from build123d import *

# Parameters (mm, degrees)
BOSS_EXTRUDE1_DEPTH = 4
BOSS_EXTRUDE2_DEPTH = 31
CHAMFER2_SIZE       = 31
CUT_EXTRUDE1_REACH  = 62.622
SKETCH3_R           = 2.75
CUT_EXTRUDE2_REACH  = 62.622
SKETCH4_R           = 2.75
CUT_EXTRUDE3_REACH  = 62.622
SKETCH5_R           = 2.75


with BuildPart() as part:
    # Sketch1 → Boss-Extrude1 (new body)
    with BuildSketch(Plane.XY):
        Polygon((0, 35), (35, 0), (35, -20), (0, -20), (0, 0), (-20, 0), (-20, 35), align=None)
    extrude(amount=BOSS_EXTRUDE1_DEPTH)

    # Sketch2 → Boss-Extrude2 (add)
    with BuildSketch(Plane.XY.offset(4)):
        Polygon((-20, 0), (0, 0), (0, -20), (4, -20), (4, -4), (35, -4), (35, 0), (4, 0), (0, 4), (0, 35), (-4, 35), (-4, 4), (-20, 4), align=None)
    extrude(amount=BOSS_EXTRUDE2_DEPTH)

    # Chamfer2
    chamfer2_edges = [part.edges().sort_by_distance(p)[0] for p in [
        (-2, 35, 35),
        (35, -2, 35),
    ]]
    chamfer(chamfer2_edges, length=CHAMFER2_SIZE)

    # Sketch3 → Cut-Extrude1 (cut, up to next)
    with BuildSketch(Plane(origin=(0, 0, 0), x_dir=(-1, 0, 0), z_dir=(0, 0, -1)), mode=Mode.PRIVATE) as cut_extrude1_sk1:
        with Locations((10, 20)):
            Circle(SKETCH3_R)
    cut_extrude1_tool1 = extrude(cut_extrude1_sk1.sketch, amount=-CUT_EXTRUDE1_REACH, mode=Mode.PRIVATE) & part.part
    # Sketch3 → Cut-Extrude1 (cut, up to next)
    with BuildSketch(Plane(origin=(0, 0, 0), x_dir=(-1, 0, 0), z_dir=(0, 0, -1)), mode=Mode.PRIVATE) as cut_extrude1_sk2:
        with Locations((-20, -10)):
            Circle(SKETCH3_R)
    cut_extrude1_tool2 = extrude(cut_extrude1_sk2.sketch, amount=-CUT_EXTRUDE1_REACH, mode=Mode.PRIVATE) & part.part
    add(cut_extrude1_tool1.solids().sort_by_distance((-10, 20, 0))[0], mode=Mode.SUBTRACT)
    add(cut_extrude1_tool2.solids().sort_by_distance((20, -10, 0))[0], mode=Mode.SUBTRACT)

    # Sketch4 → Cut-Extrude2 (cut, up to next)
    with BuildSketch(Plane.XZ, mode=Mode.PRIVATE) as cut_extrude2_sk1:
        with Locations(Location((-10, 20, 0), (0, 0, 270))):
            Circle(SKETCH4_R)
    cut_extrude2_tool1 = extrude(cut_extrude2_sk1.sketch, amount=-CUT_EXTRUDE2_REACH, mode=Mode.PRIVATE) & part.part
    add(cut_extrude2_tool1.solids().sort_by_distance((-10, 0, 20))[0], mode=Mode.SUBTRACT)

    # Sketch5 → Cut-Extrude3 (cut, up to next)
    with BuildSketch(Plane.ZY, mode=Mode.PRIVATE) as cut_extrude3_sk1:
        with Locations((20, -10)):
            Circle(SKETCH5_R)
    cut_extrude3_tool1 = extrude(cut_extrude3_sk1.sketch, amount=-CUT_EXTRUDE3_REACH, mode=Mode.PRIVATE) & part.part
    add(cut_extrude3_tool1.solids().sort_by_distance((0, -10, 20))[0], mode=Mode.SUBTRACT)


solid = part.part
Source: CAD feature listing. Evaluate the final solid. Frame: model axes, mm. A direction names the side the tool comes from. Round coordinates to 2 decimals unless told otherwise and drop trailing zeros. Loops run counter-clockwise (first coordinate to the right, second up) from the corner with the lowest first, then second, coordinate; pieces in that order, holes last. Notation, with made-up numbers: (70, 86) -> (96, 86) arc R27 cw to (96, 120) -> close; hole circle Ø10 at (-5, 76.5). An arc over 180 degrees is marked (long way). Answer as a JSON object with one key per item and string values. Group by question number.
Q1. Contact query for flat-ended pins moving along their axis: P1, Ø8, axis at x = 17.5, z = 22.5, coming from the -Y side; P2, Ø17.5, axis at y = -15.5, z = 24.5, coming from the +X side; P3, Ø10, axis at y = 10, z = 16.5, coming from the -X side; P4, Ø3.5, axis at y = -10, z = 20, coming from the +X side. Output: stop coordinate, or through.
Q2. Mould query, pull axis Y, two halves, no side actions, for faces 5 (the flat face through (16, -4, 16)), 6 (the flat face through (-14, 20, 4)), 7 (the cylindrical face through (1.972, -9.879, 17.253)). Classes: pulls with the +Y half, pulls with the -Y half, needs draft (parallel to the pull), parting line crosses it, or undercut.
Q3. Access query for faces 1 (the flat face through (20, -14, 4)), 2 (the flat face through (0, -12, 17)), 3 (the flat face through (-4, 13, 12)), 4 (the flat face through (10, 10, 4)). Directions: +Z, -Z, +X, -X, +Y, -Y. A direction counts if a zero-diameter tool reaches every point of the face in a straight line with its end or side. Return the directions, or none.
Q4. Section query B-B (y = 1). Output: boundary loops of the cut face in (x, z), plus the area to 3 significant figures.
Q5. Ray query, line 1 (Y direction, x = -10, z = 2.1); line 2 (X direction, y = 10, z = 23.5); line 3 (Z direction, x = 22, y = 9). Return the intervals inside material, ascending. Write a range as from..to.
Q6. Section query A-A (x = 20). Output: boundary loops of the cut face in (y, z).
Q7. Section query C-C (z = 20). Output: boundary loops of the cut face in (x, y).
Completed:
{
 "1": {"P1": "y = -4", "P2": "x = 4", "P3": "x = -4", "P4": "through"},
 "2": {"face 5": "pulls with the -Y half", "face 6": "needs draft", "face 7": "undercut"},
 "3": {"face 1": "+Z, +X, -Y", "face 2": "+Z, -Z, -X, -Y", "face 3": "+Z, -X, +Y", "face 4": "+Z, +X, +Y"},
 "4": {"outline": "(-20, 0) -> (34, 0) -> (34, 4) -> (3, 4) -> (3, 35) -> (-20, 35) -> close; hole circle Ø5.5 at (-10, 20)", "area": "905 mm²"},
 "5": {"line 1": "0..17.25, 22.75..35", "line 2": "-4..0", "line 3": "0..4"},
 "6": {"outline": "(-20, 0) -> (-12.75, 0) -> (-12.75, 4) -> (-20, 4) -> close; (-7.25, 0) -> (15, 0) -> (15, 4) -> (0, 4) -> (0, 19) -> (-4, 19) -> (-4, 4) -> (-7.25, 4) -> close"},
 "7": {"outline": "(-20, 0) -> (-12.75, 0) -> (-12.75, 4) -> (-20, 4) -> close; (-7.25, 0) -> (0, 0) -> (0, -7.25) -> (4, -7.25) -> (4, -4) -> (19, -4) -> (19, 0) -> (4, 0) -> (0, 4) -> (0, 19) -> (-4, 19) -> (-4, 4) -> (-7.25, 4) -> close; (0, -20) -> (4, -20) -> (4, -12.75) -> (0, -12.75) -> close"}
}
